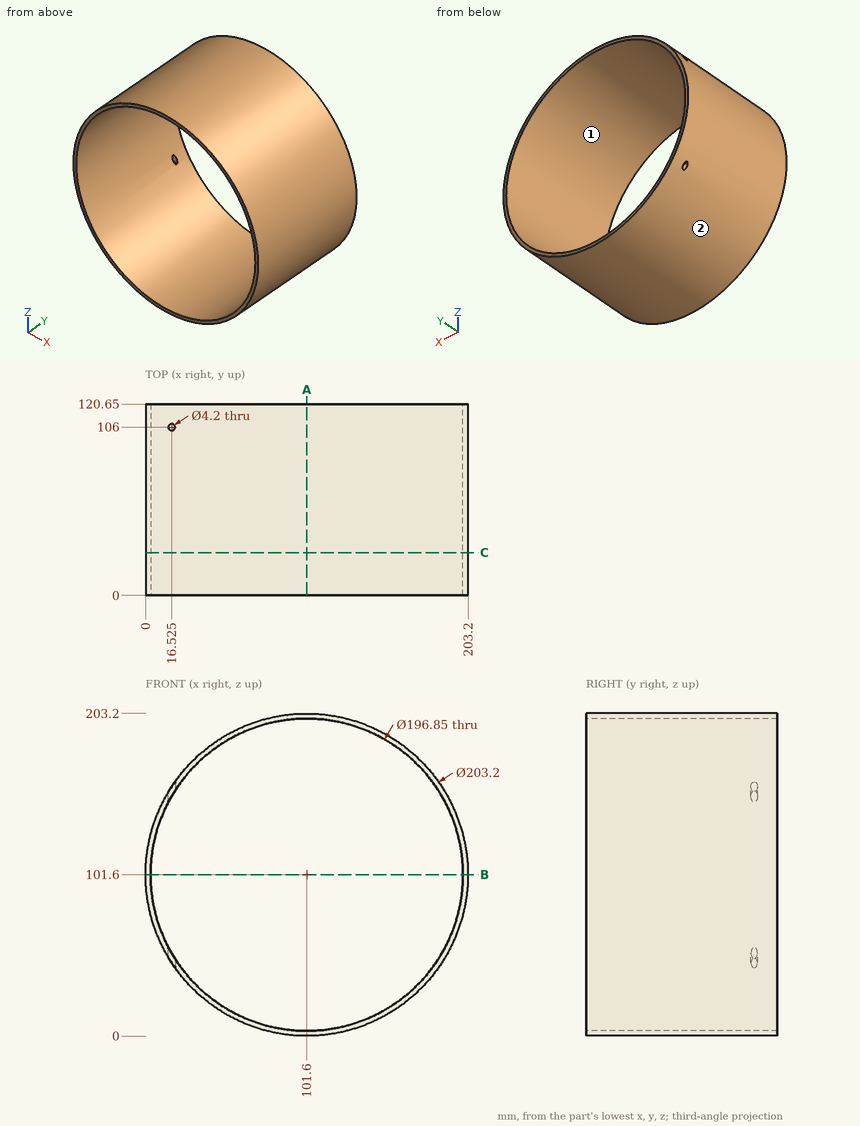
For this review, use the dimensioned drawing (mm, ordinates from the lowest corner) and the shaded views. Coordinates: 2 decimals unless noted, no trailing zeros. Loops run counter-clockwise (first coordinate to the right, second up) from the corner with the lowest first, then second, coordinate; pieces in that order, holes last.
1. Add section C-C, the plane y = 27. Give the boundary of the cut face in (x, z) (3 decimals).
2. Insertion check: P1, Ø12, axis at x = 67.5, y = 85.5, coming from the -Z side; P2, Ø12, axis at x = 80.5, y = 55.5, coming from the -Z side; P3, Ø1.5, axis at y = 39, z = 76.5, coming from the +X side. Each pin has a flat end and moves straight along its axis. Give the tip position at first contact, or say it passes through.
3. For line 1 (Z direction, x = 101.6, y = 41) (3 decimals); line 2 (X direction, y = 62, z = 101); line 3 (X direction, y = 19, z = 177.5), list the stretches that pass through material, from the lowest coordinate up.
4. Mouldability with a two-part tool opening along Z and no side actions: class the marked faces 1 and 2 as +Z half, -Z half, draft (parallel to the pull), parting line (faces both ways), or undercut.
5. Add section B-B, the plane z = 101.6. Give the boundary of the cut face in (x, y) (3 decimals).
6. Add section A-A, the plane x = 101.6. Give the boundary of the cut face in (y, z) (3 decimals), then the cut area to 3 significant figures.
Result:
1. outline: circle Ø203.2 at (101.6, 101.6); hole circle Ø196.85 at (101.6, 101.6)
2. P1: stops at z = 3.96
2. P2: stops at z = 1.13
2. P3: stops at x = 200.24
3. line 1: z = 0 to 3.175, 200.025 to 203.2
3. line 2: x = 0 to 3.18, 200.02 to 203.2
3. line 3: x = 34.06 to 38.94, 164.26 to 169.14
4. face 1: undercut
4. face 2: parting line
5. outline: (0, 0) - (3.175, 0) - (3.175, 120.65) - (0, 120.65) - close; (200.025, 0) - (203.2, 0) - (203.2, 120.65) - (200.025, 120.65) - close
6. outline: (0, 0) - (120.65, 0) - (120.65, 3.175) - (0, 3.175) - close; (0, 200.025) - (120.65, 200.025) - (120.65, 203.2) - (0, 203.2) - close
6. area: 766 mm2
